Check sheet for the modelled part. Datum: model origin and axes. Units: mm. A direction names the side the tool comes from. Round coordinates to 2 decimals unless told otherwise and drop trailing zeros. Write each loop counter-clockwise with the first axis right and the second up, starting at its lowest first coordinate (ties: lowest second). Pieces come first, ordered by that corner, then holes. Notation, with made-up numbers: (49, 62.25) -> (81, 62.25) arc R10 ccw to (81, 71.25) -> close; hole circle Ø3 at (-1, 36). An arc over 180 degrees is marked (long way). One line per item, written item: value. Start each with the question number.
```python
from build123d import *

# Parameters (mm, degrees)
SKETCH_W        = 64
SKETCH_H        = 64
PAD_DEPTH       = 2.25
SKETCH001_W     = 59
SKETCH001_H     = 59
PAD001_DEPTH    = 4.5
SKETCH002_R     = 1.5
POCKET_DEPTH    = 6.751
SKETCH003_R     = 4.25
POCKET001_DEPTH = 3
FILLET_R        = 4.5


with BuildPart() as part:
    # Sketch → Pad (new body)
    with BuildSketch(Plane.XY):
        Rectangle(SKETCH_W, SKETCH_H)
    extrude(amount=PAD_DEPTH)

    # Sketch001 (on Face6 of Pad) → Pad001 (join)
    with BuildSketch(Plane.XY.offset(2.25)):
        Rectangle(SKETCH001_W, SKETCH001_H)
    extrude(amount=PAD001_DEPTH)

    # Sketch002 → Pocket (cut, through all)
    with BuildSketch(Plane.XY):
        with Locations((-22.5, 22.5)):
            Circle(SKETCH002_R)
        with Locations((22.5, 22.5)):
            Circle(SKETCH002_R)
        with Locations((22.5, -22.5)):
            Circle(SKETCH002_R)
        with Locations((-22.5, -22.5)):
            Circle(SKETCH002_R)
    extrude(amount=POCKET_DEPTH, mode=Mode.SUBTRACT)

    # Sketch003 → Pocket001 (cut)
    with BuildSketch(Plane.XY):
        with Locations((-22.5, 22.5)):
            Circle(SKETCH003_R)
        with Locations((22.5, 22.5)):
            Circle(SKETCH003_R)
        with Locations((22.5, -22.5)):
            Circle(SKETCH003_R)
        with Locations((-22.5, -22.5)):
            Circle(SKETCH003_R)
    extrude(amount=POCKET001_DEPTH, mode=Mode.SUBTRACT)

    # Fillet
    fillet_edges = [part.edges().sort_by_distance(p)[0] for p in [
        (29.5, -29.5, 4.5),
        (32, -32, 1.125),
        (29.5, 29.5, 4.5),
        (32, 32, 1.125),
        (-29.5, -29.5, 4.5),
        (-32, -32, 1.125),
        (-29.5, 29.5, 4.5),
        (-32, 32, 1.125),
    ]]
    fillet(fillet_edges, radius=FILLET_R)


solid = part.part
```
1. Release check for a two-part mould opening along Y. For faces 6 (the face through (0, 32, 1)), 7 (the face through (-23.61, -21.49, 4.85)), 8 (the face through (0, -31, 2.25)) record: +Y half, -Y half, draft (parallel to the pull), parting line (faces both ways), or undercut.
2. Depth check by flat-ended pin: pin 1 Ø5 at (x, y) = (22.5, -22.5) entering from -Z; pin 2 Ø1.3 at (x, z) = (-9.5, 4.5) entering from +Y; pin 3 Ø1 at (y, z) = (-6, 3) entering from +X. Enter the tip coordinate at first touch or a pass-through.
3. Cross-section at B-B (y = -22.5). Record the cut outline in (x, z), plus the area to 3 significant figures.
4. Access from +Z, -Z, +X, -X, +Y, -Y to the whole of each face (thin tool, end or side, straight path). Record for faces 1 (the face through (-28.147, -28.217, 4.531)), 2 (the face through (29.5, 0, 4)), 3 (the face through (24.3, -22.4, 3)), 4 (the face through (-28.147, 28.217, 4.531)), 5 (the face through (28.217, 28.147, 4.531)).
5. Material ranges on probe 1 along Y at (x, z) = (22.5, 4.5); probe 2 along Y at (x, z) = (-22.5, 1.5), recorded low to high.
6. Cross-section at A-A (z = 1.5). Record the cut outline in (x, y).
7. Cross-section at D-D (y = 15). Record the cut outline in (x, z), plus the area to 4 significant figures.
Working result:
1. face 6: +Y half
1. face 7: undercut
1. face 8: draft
2. pin 1: stops at z = 3
2. pin 2: stops at y = 29.5
2. pin 3: stops at x = 29.5
3. outline: (-32, 0) -> (-26.75, 0) -> (-26.75, 3) -> (-24, 3) -> (-24, 6.75) -> (-29.5, 6.75) -> (-29.5, 2.25) -> (-32, 2.25) -> close; (-21, 3) -> (-18.25, 3) -> (-18.25, 0) -> (18.25, 0) -> (18.25, 3) -> (21, 3) -> (21, 6.75) -> (-21, 6.75) -> close; (24, 3) -> (26.75, 3) -> (26.75, 0) -> (32, 0) -> (32, 2.25) -> (29.5, 2.25) -> (29.5, 6.75) -> (24, 6.75) -> close
3. area: 336 mm^2
4. face 1: +Z, -X, -Y
4. face 2: +Z, +X, +Y, -Y
4. face 3: -Z
4. face 4: +Z, -X, +Y
4. face 5: +Z, +X, +Y
5. probe 1: y = -29.5 to -24, -21 to 21, 24 to 29.5
5. probe 2: y = -32 to -26.75, -18.25 to 18.25, 26.75 to 32
6. outline: (-32, -27.5) arc R4.5 ccw to (-27.5, -32) -> (27.5, -32) arc R4.5 ccw to (32, -27.5) -> (32, 27.5) arc R4.5 ccw to (27.5, 32) -> (-27.5, 32) arc R4.5 ccw to (-32, 27.5) -> close; hole circle Ø8.5 at (-22.5, -22.5); hole circle Ø8.5 at (-22.5, 22.5); hole circle Ø8.5 at (22.5, -22.5); hole circle Ø8.5 at (22.5, 22.5)
7. outline: (-32, 0) -> (32, 0) -> (32, 2.25) -> (29.5, 2.25) -> (29.5, 6.75) -> (-29.5, 6.75) -> (-29.5, 2.25) -> (-32, 2.25) -> close
7. area: 409.5 mm^2
